Model file for the job. Use its own axes, mm. Round coordinates to 2 decimals unless told otherwise and drop trailing zeros. Order: outer loops, then holes, each group sorted by start corner. A loop starts at its lowest first (then second) coordinate and runs counter-clockwise, first axis right, second up. Notation, with made-up numbers: (-11.75, 82) -> (25.25, 82) arc R13 ccw to (25.25, 99) -> close; hole circle Ø11 at (-18.75, 39). An arc over 180 degrees is marked (long way). Use CSV: the item, a comma, the result in double quotes.
Autodesk Inventor part; units mm, degrees
ref_plane "YZ Plane" through (0, 0, 0) normal (1, 0, 0) x (0, 1, 0)
ref_plane "XZ Plane" through (0, 0, 0) normal (0, 1, 0) x (-1, 0, 0)
ref_plane "XY Plane" through (0, 0, 0) normal (0, 0, 1) x (1, 0, 0)
sketch "Sketch2" plane through (0, 0, 0) normal (0, 1, 0) x (-1, 0, 0)
  line L0 (0, 0) -> (-24.2467, -24.2467) construction
  line L1 (0, 0) -> (-34.29, 0) construction
  circle A0 centre (-24.2467, -24.2467) radius 119.0625
  dimension "d6" = 34.29
  dimension "d7" = 315
  dimension "d8" = 238.125
extrude "Extrusion1" add sketch "Sketch2" against normal blind 6.35
sketch "Sketch1" plane through (0, 0, 0) normal (0, 1, 0) x (-1, 0, 0)
  line L0 (0, 0) -> (-64.6578, -64.6578) construction
  line L1 (0, 0) -> (91.44, 0) construction
  circle A0 centre (-64.6578, -64.6578) radius 48.26
  line L2 (0, 0) -> (40.4112, 40.4112) construction
  line L3 (0, 0) -> (57.15, 0) construction
  circle A1 centre (40.4112, 40.4112) radius 13.97
  dimension "d0" = 91.44
  dimension "d1" = 135
  dimension "d2" = 96.52
  dimension "d3" = 57.15
  dimension "d4" = 45
  dimension "d5" = 27.94
extrude "Extrusion2" cut sketch "Sketch1" against normal up to surface (6.35 mm away)
sketch "Sketch9" plane through (24.2467, 0, -24.2467) normal (0, 1, 0) x (1, 0, 0)
  circle A0 centre (40.4112, 40.4112) radius 48.26
  circle A1 centre (-64.6578, -64.6578) radius 13.97
  line L0 (40.4112, 40.4112) -> (-64.6578, -64.6578)
  circle A2 centre (-29.6348, -29.6348) radius 63.5
  circle A3 centre (29.6348, 29.6348) radius 63.5
  circle A4 centre (40.4112, 40.4112) radius 48.26
  line L1 (-33.7328, 33.7328) -> (33.7328, -33.7328)
  point P0 (-24.2467, -24.2467)
  dimension "d81" = 127
  dimension "d82" = 127
sketch "Sketch10" plane through (24.2467, 0, -24.2467) normal (0, 1, 0) x (1, 0, 0)
  circle A0 centre (0, 0) radius 119.0625
  circle A1 centre (0, 0) radius 101.6 construction
  line L0 (0, 0) -> (0, 101.6) construction
  line L1 (0, 0) -> (-101.6, 0) construction
  line L2 (0, 0) -> (0, -101.6) construction
  line L3 (0, 0) -> (101.6, 0) construction
  point P0 (-24.2467, -24.2467)
  dimension "d83" = 203.2
  dimension "d86" = 360
hole "Hole4" at (-77.3533, 0, -24.2467) at (125.8467, 0, -24.2467) at (24.2467, 0, 77.3533) at (24.2467, 0, -125.8467) direction (0, -1, 0) diameter 6.7564 end through all
sketch "Sketch11" plane through (24.2467, 0, -24.2467) normal (0, 1, 0) x (1, 0, 0)
  line L0 (117.2853, -50.0358) -> (124.9604, -50.0358)
  line L1 (124.9604, -50.0358) -> (124.9604, 67.1373)
  line L2 (124.9604, 67.1373) -> (117.2853, 67.1373)
  line L3 (117.2853, 67.1373) -> (117.2853, -50.0358)
  line L4 (0, 0) -> (82.6418, -82.6418)
  line L5 (0, 0) -> (116.8732, 0) construction
  line L6 (82.6418, -82.6418) -> (56.0171, -109.2666)
  line L7 (56.0171, -109.2666) -> (65.8131, -119.0625)
  line L8 (65.8131, -119.0625) -> (121.1228, -63.7527)
  line L9 (121.1228, -63.7527) -> (111.3269, -53.9568)
  line L10 (111.3269, -53.9568) -> (82.6418, -82.6418)
  point P0 (-24.2467, -24.2467)
  dimension "d95" = 45
extrude "Extrusion3" cut sketch "Sketch11" against normal blind 44.45
properties part number "2K8 stage mini" material "Copper"
Q1. Cut at A-A (x = 100). Give the cut face in (y, z).
From the geometry:
outline,"(-6.35, -116.1) -> (0, -116.1) -> (0, -97.52) -> (-6.35, -97.52) -> close; (-6.35, -31.8) -> (0, -31.8) -> (0, 65.28) -> (-6.35, 65.28) -> close"
Q2. Pin check, flat tips, straight feed: pin 1 (17 mm diameter, centred on x = -40.41, z = 40.41, fed in from -Y); pin 2 (2 mm diameter, centred on y = -5, z = -111.5, fed in from +X). Stop position of each tip, or through.
From the geometry:
pin 1,"passes through"
pin 2,"stops at x = 106.32"
Q3. Probe line 1 along Z through (x, y) = (-31.5, -1.25); line 2 along Z through (x, y) = (-76, -5); line 3 along Z through (x, y) = (25, -5.25). List the from-to ranges inside material, lowest first.
From the geometry:
line 1,"z = -129.45 to 29.65, 51.17 to 80.96"
line 2,"z = -88.48 to -27.34, -21.15 to 39.99"
line 3,"z = -143.31 to -129.14, -122.55 to -92.16, -37.16 to 74.06, 80.65 to 94.81"
Q4. Cut at B-B (z = -53.5). Give the cut face in (x, y), plus the area to 3 significant figures.
From the geometry:
outline,"(-91.17, -6.35) -> (17.71, -6.35) -> (17.71, 0) -> (-91.17, 0) -> close; (111.61, -6.35) -> (139.66, -6.35) -> (139.66, 0) -> (111.61, 0) -> close"
area,"869 mm²"
Q5. Mould opens along X. For faces 1 (the cylindrical face through (122.5, -3.2, -24.7)), 2 (the flat face through (141.532, -3, -25)), 3 (the cylindrical face through (-83.57, -3.13, -74.76)), 4 (the flat face through (25, 0, -23)) say: +X half, -X half, draft (parallel to the pull), parting line (faces both ways), or undercut.
From the geometry:
face 1,"undercut"
face 2,"+X half"
face 3,"parting line"
face 4,"draft"
Q6. Cut at C-C (y = -3.75). Give the cut face in (x, z) (1 decimal), plus the area to 3 significant figures.
From the geometry:
outline,"(90.8, 74.5) arc R119.1 ccw (long way) to (141.5, -44.7) -> (141.5, -3.8) arc R119.1 ccw to (123, 42.3) -> (106.9, 58.4) -> close; hole circle Ø6.8 at (-77.4, -24.2); hole circle Ø27.9 at (-40.4, 40.4); hole circle Ø96.5 at (64.7, -64.7); hole circle Ø6.8 at (24.2, -125.8); hole circle Ø6.8 at (24.2, 77.4); hole circle Ø6.8 at (125.8, -24.2)"
area,"36,300 mm²"
Q7. Cut at D-D (z = 22.5). Give the cut face in (x, y), plus the area to 3 significant figures.
From the geometry:
outline,"(-85.26, -6.35) -> (133.75, -6.35) -> (133.75, 0) -> (-85.26, 0) -> close"
area,"1,390 mm²"
